Input: part model. Units: mm. Frame: model coordinates. A direction names the side the tool comes from. Give positions to 0.01 mm unless a question says otherwise; leave off trailing zeros. Order: outer loops, then holes, each group sorted by start corner. A loop starts at its lowest first (then second) coordinate and runs counter-clockwise, first axis right, second up. Notation, with made-up numbers: (11, 42) - (35, 42) arc R18 ccw to (35, 61) - close; hole circle Ø8 at (-9.75, 36). An arc over 180 degrees is marked (long way). Answer in a Markdown table with one row per item. Add a question column.
from build123d import *

# Parameters (mm, degrees)
BOSS_EXTRUDE1_DEPTH = 9.525
SKETCH2_R           = 6.35
CUT_EXTRUDE1_DEPTH  = 83.55
FILLET1_R           = 1.27
HOLE1_D             = 7.94512
HOLE1_DEPTH         = 46.0375
HOLE1_TIP           = 2.386954861


with BuildPart() as part:
    # Sketch1 → Boss-Extrude1 (new body, symmetric)
    with BuildSketch(Plane.XY):
        Polygon((4.7625, 0), (-4.7625, 0), (-4.7625, 38.1), (-41.275, 38.1), (-41.275, 171.45), (-27.051, 171.45), (-27.051, 158.75), (-28.575, 158.75), (-28.575, 47.625), (28.575, 47.625), (28.575, 158.75), (27.051, 158.75), (27.051, 171.45), (41.275, 171.45), (41.275, 38.1), (4.7625, 38.1), align=None)
    extrude(amount=BOSS_EXTRUDE1_DEPTH, both=True)

    # Sketch2 → Cut-Extrude1 (cut, through all)
    with BuildSketch(Plane.ZY.offset(41.275)):
        with Locations((0, 76.2)):
            Circle(SKETCH2_R)
        with Locations((0, 139.7)):
            Circle(SKETCH2_R)
    extrude(amount=-CUT_EXTRUDE1_DEPTH, mode=Mode.SUBTRACT)

    # Fillet1
    fillet1_edges = [part.edges().sort_by_distance(p)[0] for p in [
        (4.7625, 0, 0),
        (-4.7625, 0, 0),
        (-28.575, 158.75, 0),
        (-28.575, 47.625, 0),
        (28.575, 47.625, 0),
        (28.575, 158.75, 0),
    ]]
    fillet(fillet1_edges, radius=FILLET1_R)

    # Hole1
    with Locations(Plane(origin=(4.7625, 0, 0), x_dir=(0, 0, 1), z_dir=(1, 0, 0))):
        with Locations((0, -25.4), (0, -10.16)):
            Hole(HOLE1_D / 2, depth=HOLE1_DEPTH)
            with Locations((0, 0, -(HOLE1_DEPTH + HOLE1_TIP / 2))):  # 118° drill point
                Cone(0, HOLE1_D / 2, HOLE1_TIP, mode=Mode.SUBTRACT)


solid = part.part
Q1. Section D-D, the plane x = -13. Return loops of the section in (y, z) (3 decimals), then the cut area to 3 significant figures.
Q2. Section B-B, the plane y = 107.5. Return loops of the section in (x, z) (3 decimals).
Q3. Pull-direction query (Z, two-part tool) for faces 5 (the flat face through (-30, 92, -9.525)), 6 (the flat face through (34, 171.45, 0)), 7 (the cylindrical face through (-35.01, 133.5, -1.38)); classes: +Z half, -Z half, draft (parallel to the pull), parting line (faces both ways), or undercut.
Q4. Access query for faces 1 (the flat face through (-28.575, 104, 0)), 2 (the flat face through (27.051, 165, 0)), 3 (the flat face through (23, 38.1, 0)), 4 (the flat face through (-4.762, 19, 0)). Directions: +Z, -Z, +X, -X, +Y, -Y. A direction counts if a zero-diameter tool reaches every point of the face in a straight line with its end or side. Return the directions, or none.
Q5. Contact query for flat-ended pins moving along their axis: P1, Ø1, axis at x = 28, y = 99.5, coming from the +Z side; P2, Ø5.5, axis at y = 22, z = -2, coming from the +X side; P3, Ø1.5, axis at x = -6.5, z = 4, coming from the -Y side; P4, Ø9, axis at y = 10.16, z = 0, coming from the -X side. Output: stop coordinate, or through.
Q6. Section C-C, the plane z = 0. State how many separate pieces and enclosed holes the cut face has, then the cut area to 3 significant figures.
Q7. Line query: probe 1 along Y at (x, z) = (-2.25, 0) (3 decimals); probe 2 along Y at (x, z) = (-32.5, 0); probe 3 along X at (y, z) = (85, 3.75) (3 decimals). Output: solid intervals per line, ascending.
Q8. Section A-A, the plane y = 76.2. Return loops of the section in (x, z) (3 decimals), then the cut area to 3 significant figures.
Computed:
| question | item | result |
|---|---|---|
| 1 | outline | (38.1, -9.525) - (47.625, -9.525) - (47.625, 9.525) - (38.1, 9.525) - close |
| 1 | area | 181 mm^2 |
| 2 | outline | (-41.275, -9.525) - (-28.575, -9.525) - (-28.575, 9.525) - (-41.275, 9.525) - close; (28.575, -9.525) - (41.275, -9.525) - (41.275, 9.525) - (28.575, 9.525) - close |
| 3 | face 5 | -Z half |
| 3 | face 6 | draft |
| 3 | face 7 | undercut |
| 4 | face 1 | +Z, -Z |
| 4 | face 2 | +Z, -Z, +Y |
| 4 | face 3 | +Z, -Z, +X, -Y |
| 4 | face 4 | +Z, -Z, -X, -Y |
| 5 | P1 | passes through |
| 5 | P2 | stops at x = 4.76 |
| 5 | P3 | stops at y = 38.1 |
| 5 | P4 | stops at x = -4.76 |
| 6 | separate pieces | 7 |
| 6 | enclosed holes | 0 |
| 6 | area | 3,540 mm^2 |
| 7 | probe 1 | y = 0 to 6.187, 14.133 to 21.427, 29.373 to 47.625 |
| 7 | probe 2 | y = 38.1 to 69.85, 82.55 to 133.35, 146.05 to 171.45 |
| 7 | probe 3 | x = -41.275 to -28.575, 28.575 to 41.275 |
| 8 | outline | (-41.275, -9.525) - (-28.575, -9.525) - (-28.575, -6.35) - (-41.275, -6.35) - close; (-41.275, 6.35) - (-28.575, 6.35) - (-28.575, 9.525) - (-41.275, 9.525) - close; (28.575, -9.525) - (41.275, -9.525) - (41.275, -6.35) - (28.575, -6.35) - close; (28.575, 6.35) - (41.275, 6.35) - (41.275, 9.525) - (28.575, 9.525) - close |
| 8 | area | 161 mm^2 |
